Here's the drawing with two shaded views (mm, measured from the low corner). I have some questions. A direction names the side the tool comes from. Round coordinates to 2 decimals unless told otherwise and drop trailing zeros. Write each loop counter-clockwise with the first axis right and the second up, starting at its lowest first coordinate (ties: lowest second). Pieces come first, ordered by that corner, then holes. Notation, with made-up numbers: (-23, 73) -> (-6, 73) arc R23 ccw to (-6, 109) -> close; hole circle Ø1 at (-20.75, 44). An arc over 180 degrees is marked (long way). Use CSV: the item, a comma, the result in double quotes.
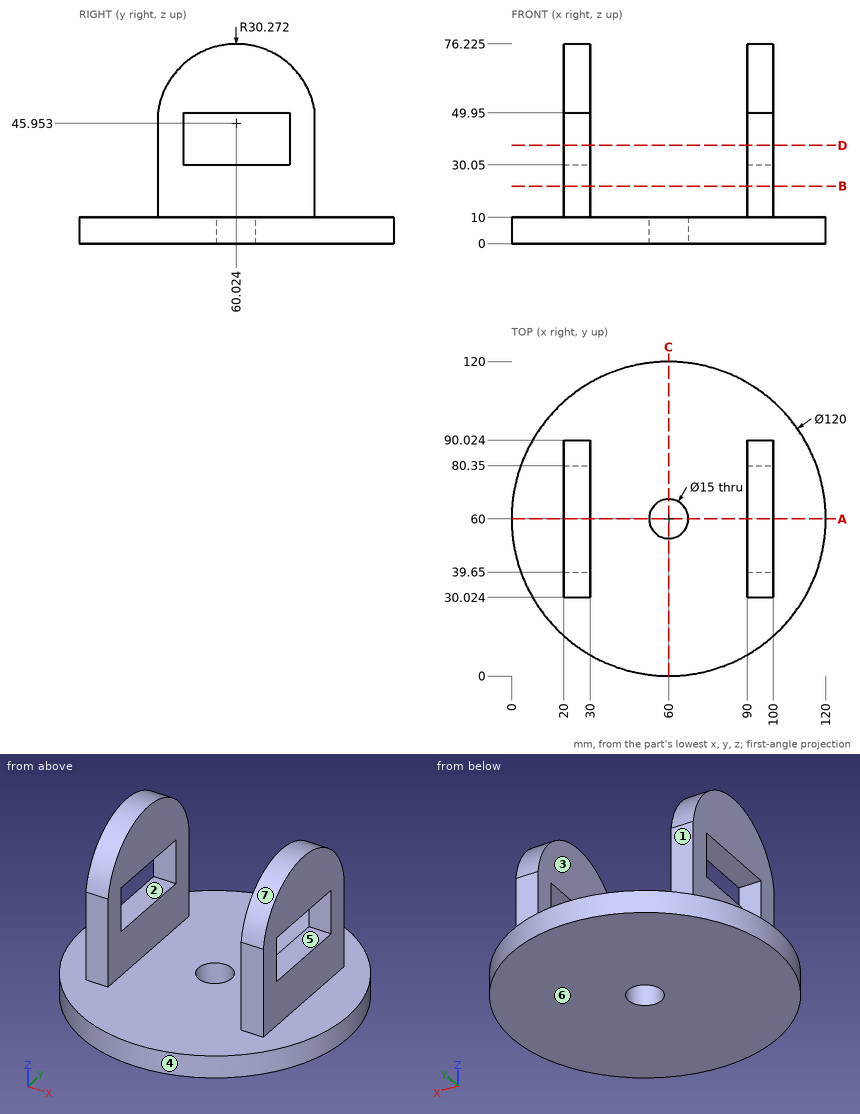
Q1. If we mould it in two halves opening along Z, with no side actions, what happens to the marked faces 4, 5, 6 and 7? For each: released by +Z, released by -Z, zero draft, split by the parting line, or undercut.
Resolved:
face 4,"zero draft"
face 5,"undercut"
face 6,"released by -Z"
face 7,"released by +Z"
Q2. Suppose I cut it at A-A (y = 60). Count the separate pieces of the cut face and the enclosed holes in it, and give its area (3 significant figures).
Resolved:
separate pieces,"4"
enclosed holes,"0"
area,"1,980 mm^2"
Q3. On a 3-axis mill with a long thin cutter (end or side, diameter ignored), from which of +Z, -Z, +X, -X, +Y, -Y can I reach the whole of each face in a straight line? I mean the marked faces 1, 2 and 3. Say none if no direction works.
Resolved:
face 1,"+Z, +X, -X, +Y"
face 2,"+X, -X"
face 3,"+Z, +Y, -Y"
Q4. Suppose I cut it at C-C (x = 60). Write out the boundary of the cut face in (y, z).
Resolved:
outline,"(0, 0) -> (52.5, 0) -> (52.5, 10) -> (0, 10) -> close; (67.5, 0) -> (120, 0) -> (120, 10) -> (67.5, 10) -> close"
Q5. Will these pins go through, and if not, where does the flat tip stop? P1, Ø11, axis at x = 22.5, y = 53.5, coming from the +Z side; P2, Ø3, axis at x = 97, y = 52.5, coming from the +Z side; P3, Ø18, axis at y = 58, z = 55.5, coming from the -X side.
Resolved:
P1,"stops at z = 76.21"
P2,"stops at z = 75.62"
P3,"stops at x = 20"
Q6. Suppose I cut it at D-D (z = 37.5). Write out the boundary of the cut face in (x, y).
Resolved:
outline,"(20, 30.02) -> (30, 30.02) -> (30, 39.65) -> (20, 39.65) -> close; (20, 80.35) -> (30, 80.35) -> (30, 90.02) -> (20, 90.02) -> close; (90, 30.02) -> (100, 30.02) -> (100, 39.65) -> (90, 39.65) -> close; (90, 80.35) -> (100, 80.35) -> (100, 90.02) -> (90, 90.02) -> close"
Q7. Suppose I cut it at B-B (z = 22). Write out the boundary of the cut face in (x, y).
Resolved:
outline,"(20, 30.02) -> (30, 30.02) -> (30, 90.02) -> (20, 90.02) -> close; (90, 30.02) -> (100, 30.02) -> (100, 90.02) -> (90, 90.02) -> close"
Q8. Please list where these lines run through material, in increasing order: probe 1 along Y at (x, z) = (60, 3.25); probe 2 along X at (y, z) = (50.5, 52); probe 3 along Z at (x, y) = (54.5, 90).
Resolved:
probe 1,"y = 0 to 52.5, 67.5 to 120"
probe 2,"x = 20 to 30, 90 to 100"
probe 3,"z = 0 to 10"
